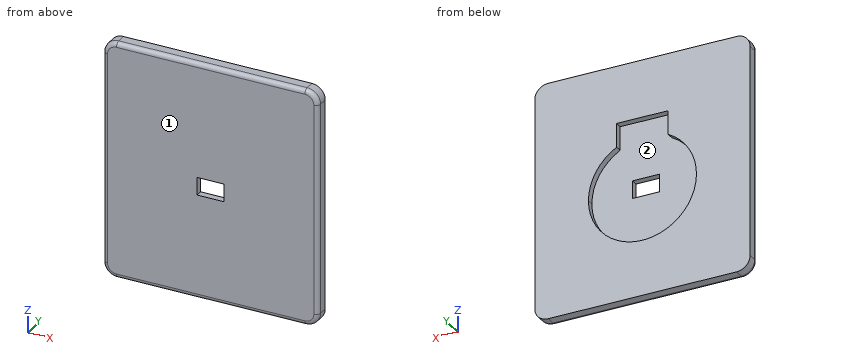
```python
from build123d import *

# Parameters (mm, degrees)
SKETCH1_W           = 42
SKETCH1_H           = 47.5
BOSS_EXTRUDE1_DEPTH = 3
CUT_EXTRUDE2_DEPTH  = 1.5
SKETCH3_W           = 6
SKETCH3_H           = 4
CUT_EXTRUDE3_DEPTH  = 5
SKETCH4_W           = 48
SKETCH4_H           = 53.5
SKETCH4_W_2         = 42
SKETCH4_H_2         = 47.5
BOSS_EXTRUDE2_DEPTH = 3
FILLET1_R           = 3
FILLET2_R           = 1


with BuildPart() as part:
    # Sketch1 → Boss-Extrude1 (new body)
    with BuildSketch(Plane(origin=(0, 0, 0), x_dir=(1, 0, 0), z_dir=(0, 1, 0))):
        Rectangle(SKETCH1_W, SKETCH1_H)
    extrude(amount=BOSS_EXTRUDE1_DEPTH)

    # Sketch2 → Cut-Extrude2 (cut)
    with BuildSketch(Plane(origin=(0, 3, 0), x_dir=(1, 0, 0), z_dir=(0, 1, 0))):
        with BuildLine():
            ThreePointArc((12.038461538, 2.211538462), (-6.152373622, 12.559139876), (-5.75, -8.364947543))
            Line((-5.75, -8.364947543), (-5.75, -7.75))
            Line((-5.75, -7.75), (5.75, -7.75))
            Line((5.75, -7.75), (5.75, -8.364947543))
            ThreePointArc((5.75, -8.364947543), (10.347601414, -3.94083516), (12.038461538, 2.211538462))
        make_face()
        with BuildLine():
            Line((-5.75, -7.75), (-5.75, -8.364947543))
            ThreePointArc((-5.75, -8.364947543), (0, -9.826923077), (5.75, -8.364947543))
            Line((5.75, -8.364947543), (5.75, -7.75))
            Line((5.75, -7.75), (-5.75, -7.75))
        make_face()
        with BuildLine():
            Line((-5.75, -8.364947543), (-5.75, -13.75))
            Line((-5.75, -13.75), (5.75, -13.75))
            Line((5.75, -13.75), (5.75, -8.364947543))
            ThreePointArc((5.75, -8.364947543), (0, -9.826923077), (-5.75, -8.364947543))
        make_face()
    extrude(amount=-CUT_EXTRUDE2_DEPTH, mode=Mode.SUBTRACT)

    # Sketch3 → Cut-Extrude3 (cut)
    with BuildSketch(Plane(origin=(0, 3, 0), x_dir=(1, 0, 0), z_dir=(0, 1, 0))):
        with Locations((0, 1.25)):
            Rectangle(SKETCH3_W, SKETCH3_H)
    extrude(amount=-CUT_EXTRUDE3_DEPTH, mode=Mode.SUBTRACT)

    # Sketch4 → Boss-Extrude2 (add)
    with BuildSketch(Plane(origin=(0, 0, 0), x_dir=(1, 0, 0), z_dir=(0, 1, 0))):
        Rectangle(SKETCH4_W, SKETCH4_H)
        Rectangle(SKETCH4_W_2, SKETCH4_H_2, mode=Mode.SUBTRACT)
    extrude(amount=BOSS_EXTRUDE2_DEPTH)

    # Fillet1
    fillet1_edges = [part.edges().sort_by_distance(p)[0] for p in [
        (-24, 1.5, -26.75),
        (-24, 1.5, 26.75),
        (24, 1.5, 26.75),
        (24, 1.5, -26.75),
    ]]
    fillet(fillet1_edges, radius=FILLET1_R)

    # Fillet2
    fillet2_edges = [part.edges().sort_by_distance(p)[0] for p in [
        (-24, 0, 0),
        (0, 0, -26.75),
        (24, 0, 0),
        (0, 0, 26.75),
        (-23.121320344, 0, 25.871320344),
        (23.121320344, 0, 25.871320344),
        (23.121320344, 0, -25.871320344),
        (-23.121320344, 0, -25.871320344),
    ]]
    fillet(fillet2_edges, radius=FILLET2_R)


solid = part.part
```
The listing builds one solid part. Answer for the finished solid, in the listing's coordinates (mm). Face numbers are marked on the shaded views. Give positions to 0.01 mm unless a question says otherwise; leave off trailing zeros. Write each loop counter-clockwise with the first axis right and the second up, starting at its lowest first coordinate (ties: lowest second). Pieces come first, ordered by that corner, then holes. Notation, with made-up numbers: (3.25, -35.75) -> (41.25, -35.75) arc R20 ccw to (41.25, -12.75) -> close; hole circle Ø7 at (14, 77). An arc over 180 degrees is marked (long way). Use one line per item in the form item = value.
1) Section A-A on x = 0 is taken. Write down the section's boundary in (y, z), plus the area to 3 significant figures.
Result:
outline = (0, -25.75) arc R1 ccw to (1, -26.75) -> (3, -26.75) -> (3, -14.25) -> (1.5, -14.25) -> (1.5, -3.25) -> (0, -3.25) -> close; (0, 0.75) -> (1.5, 0.75) -> (1.5, 13.75) -> (3, 13.75) -> (3, 26.75) -> (1, 26.75) arc R1 ccw to (0, 25.75) -> close
area = 112 mm²
2) For a pull along X with two mould halves and no side action, classify the marked faces 1 and 2 as +X half, -X half, draft (parallel to the pull), parting line (faces both ways), or undercut.
Result:
face_1 = draft
face_2 = undercut
3) This flat-tipped pin is pushed along its axis until it touches: P1, Ø19.5, axis at x = 2, z = -2, coming from the +Y side. Where does it stop, or does it pass through?
Result:
P1 = 1.5
4) Section D-D on x = -11 is taken. Write down the section's boundary in (y, z).
Result:
outline = (0, -25.75) arc R1 ccw to (1, -26.75) -> (3, -26.75) -> (3, -7.1) -> (1.5, -7.1) -> (1.5, 2.68) -> (3, 2.68) -> (3, 26.75) -> (1, 26.75) arc R1 ccw to (0, 25.75) -> close
5) Section B-B on y = 2.1 is taken. Write down the section's boundary in (x, z), plus the area to 3 significant figures.
Result:
outline = (-24, -23.75) arc R3 ccw to (-21, -26.75) -> (21, -26.75) arc R3 ccw to (24, -23.75) -> (24, 23.75) arc R3 ccw to (21, 26.75) -> (-21, 26.75) arc R3 ccw to (-24, 23.75) -> close; hole (-5.75, 8.36) arc R12.04 ccw (long way) to (5.75, 8.36) -> (5.75, 13.75) -> (-5.75, 13.75) -> close
area = 2,050 mm²
6) Straight lines are drawn through the part: probe 1 along Z at (x, y) = (0, 2.45); probe 2 along Y at (x, z) = (9, -7.5); probe 3 along Z at (x, y) = (10, 2.45). For each, find the intervals that lie inside material, in ascending order.
Result:
probe_1 = -26.75 to -14.25, 13.75 to 26.75
probe_2 = 0 to 1.5
probe_3 = -26.75 to -8.91, 4.49 to 26.75
7) Section C-C on z = 10 is taken. Write down the section's boundary in (x, y), plus the area to 3 significant figures.
Result:
outline = (-24, 1) arc R1 ccw to (-23, 0) -> (23, 0) arc R1 ccw to (24, 1) -> (24, 3) -> (5.75, 3) -> (5.75, 1.5) -> (-5.75, 1.5) -> (-5.75, 3) -> (-24, 3) -> close
area = 126 mm²
